Can you work these out from the drawing? Everything is in mm from the part's minimum corner. A direction names the side the tool comes from. Coordinates: 2 decimals unless noted, no trailing zeros. Loops run counter-clockwise (first coordinate to the right, second up) from the corner with the lowest first, then second, coordinate; pieces in that order, holes last.
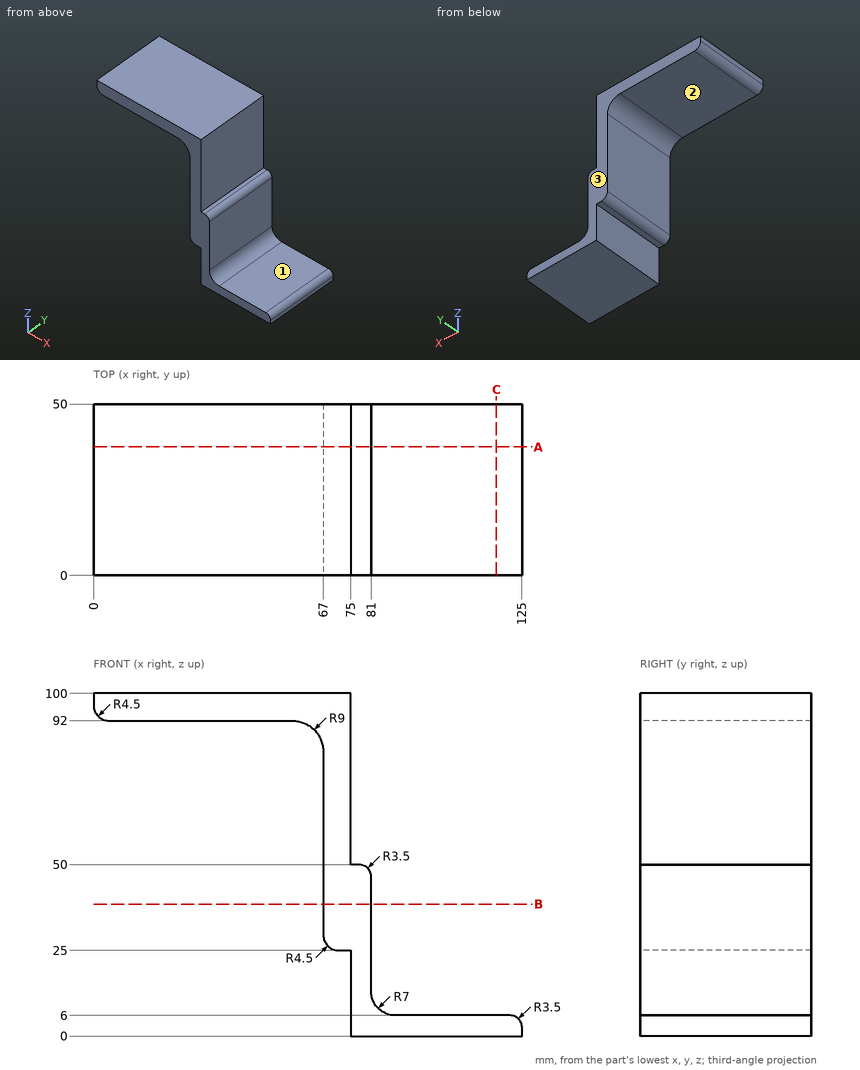
1) For the marked faces 1, 2 and 3, which set-ups out of +Z, -Z, +X, -X, +Y, -Y let a thin tool reach every point of the face, with its end or its side?
2) Will these pins go through, and if not, where does the flat tip stop? pin 1 (5 mm diameter, centred on x = 48.5, y = 10, fed in from -Z); pin 2 (4 mm diameter, centred on y = 35.5, z = 40.5, fed in from -X); pin 3 (0.8 mm diameter, centred on x = 77, y = 33, fed in from +Z).
3) If I drill on L1, parallel to X at y = 26, z = 16; L2, parallel to Z at x = 55, y = 9; L3, parallel to X at y = 31.5, z = 74.5, over which ranges is the centre line in solid material (lowest first)?
4) Imagine slicing it at C-C on x = 117.5. List the corners of the cut face in (y, z) for me.
5) Imagine slicing it at B-B on z = 38.5. List the corners of the cut face in (x, y) for me, plus the area to 3 significant figures.
6) Imagine slicing it at A-A on y = 37.5. List the corners of the cut face in (x, z) for me, plus the area to 3 significant figures.
Solved:
1. face 1: +Z, +X, +Y, -Y
1. face 2: -Z, -X, +Y, -Y
1. face 3: +Z, -Z, +X, -X, +Y
2. pin 1: stops at z = 92
2. pin 2: stops at x = 67
2. pin 3: stops at z = 50
3. L1: x = 75 to 81
3. L2: z = 92 to 100
3. L3: x = 67 to 75
4. outline: (0, 0) - (50, 0) - (50, 6) - (0, 6) - close
5. outline: (67, 0) - (81, 0) - (81, 50) - (67, 50) - close
5. area: 700 mm2
6. outline: (0, 96.5) arc R4.5 ccw to (4.5, 92) - (58, 92) arc R9 cw to (67, 83) - (67, 29.5) arc R4.5 ccw to (71.5, 25) - (75, 25) - (75, 0) - (125, 0) - (125, 2.5) arc R3.5 ccw to (121.5, 6) - (88, 6) arc R7 cw to (81, 13) - (81, 46.5) arc R3.5 ccw to (77.5, 50) - (75, 50) - (75, 100) - (0, 100) - close
6. area: 1,710 mm2
